from build123d import *

# Parameters (mm, degrees)
SKETCH1_W           = 93.5
SKETCH1_H           = 123
SKETCH1_R           = 6
SKETCH1_W_2         = 57.5
SKETCH1_H_2         = 30
BOSS_EXTRUDE1_DEPTH = 6
SKETCH2_R           = 4.5
SKETCH2_R_2         = 2.1
BOSS_EXTRUDE2_DEPTH = 3
CHAMFER2_SIZE       = 5
SKETCH5_R           = 2.875
CUT_EXTRUDE2_DEPTH  = 3
SKETCH6_R           = 1.625
CUT_EXTRUDE3_DEPTH  = 23
SKETCH7_W           = 5
SKETCH7_H           = 12
SKETCH7_W_2         = 8
SKETCH7_H_2         = 24.8
SKETCH7_R           = 2.1
BOSS_EXTRUDE3_DEPTH = 6
CHAMFER3_SIZE       = 3
CHAMFER3_SIZE2      = 5.196152423
SKETCH9_R           = 2.1
CUT_EXTRUDE5_DEPTH  = 3


with BuildPart() as part:
    # Sketch1 → Boss-Extrude1 (new body)
    with BuildSketch(Plane.XY):
        with Locations((0, 28.5)):
            Rectangle(SKETCH1_W, SKETCH1_H)
        with Locations((0, 60)):
            Circle(SKETCH1_R, mode=Mode.SUBTRACT)
        Rectangle(SKETCH1_W_2, SKETCH1_H_2, mode=Mode.SUBTRACT)
    extrude(amount=BOSS_EXTRUDE1_DEPTH)

    # Sketch2 → Boss-Extrude2 (add)
    # profile 1 of 4: a face of its own
    with BuildSketch(Plane(origin=(0, 0, 0), x_dir=(-1, 0, 0), z_dir=(0, 0, -1))):
        with Locations((34, 21.75)):
            Circle(SKETCH2_R)
        with Locations((34, 21.75)):
            Circle(SKETCH2_R_2, mode=Mode.SUBTRACT)
    # profile 2 of 4: a face of its own
    with BuildSketch(Plane(origin=(0, 0, 0), x_dir=(-1, 0, 0), z_dir=(0, 0, -1))):
        with Locations((-34, -17.25)):
            Circle(SKETCH2_R)
        with Locations((-34, -17.25)):
            Circle(SKETCH2_R_2, mode=Mode.SUBTRACT)
    # profile 3 of 4: a face of its own
    with BuildSketch(Plane(origin=(0, 0, 0), x_dir=(-1, 0, 0), z_dir=(0, 0, -1))):
        with Locations((34, -17.25)):
            Circle(SKETCH2_R)
        with Locations((34, -17.25)):
            Circle(SKETCH2_R_2, mode=Mode.SUBTRACT)
    # profile 4 of 4: a face of its own
    with BuildSketch(Plane(origin=(0, 0, 0), x_dir=(-1, 0, 0), z_dir=(0, 0, -1))):
        with Locations((-34, 21.75)):
            Circle(SKETCH2_R)
        with Locations((-34, 21.75)):
            Circle(SKETCH2_R_2, mode=Mode.SUBTRACT)
    extrude(amount=BOSS_EXTRUDE2_DEPTH)

    # Chamfer2
    chamfer2_edges = [part.edges().sort_by_distance(p)[0] for p in [
        (-46.75, 90, 3),
        (46.75, 90, 3),
        (46.75, -33, 3),
        (-46.75, -33, 3),
    ]]
    chamfer(chamfer2_edges, length=CHAMFER2_SIZE)

    # Sketch5 → Cut-Extrude2 (cut)
    with BuildSketch(Plane.XY.offset(6)):
        with Locations((39.25, -25.5)):
            Circle(SKETCH5_R)
        with Locations((39.25, 82.5)):
            Circle(SKETCH5_R)
        with Locations(Location((-39.25, -25.5, 0), (0, 0, 180))):
            Circle(SKETCH5_R)
        with Locations(Location((-39.25, 82.5, 0), (0, 0, 180))):
            Circle(SKETCH5_R)
    extrude(amount=-CUT_EXTRUDE2_DEPTH, mode=Mode.SUBTRACT)

    # Sketch6 → Cut-Extrude3 (cut)
    with BuildSketch(Plane.XY.offset(3)):
        with Locations((39.25, -25.5)):
            Circle(SKETCH6_R)
        with Locations((-39.25, -25.5)):
            Circle(SKETCH6_R)
        with Locations((-39.25, 82.5)):
            Circle(SKETCH6_R)
        with Locations((39.25, 82.5)):
            Circle(SKETCH6_R)
    extrude(amount=-CUT_EXTRUDE3_DEPTH, mode=Mode.SUBTRACT)

    # Sketch7 → Boss-Extrude3 (add)
    # profile 1 of 2: a face of its own
    with BuildSketch(Plane.XY):
        with Locations((-8, 60)):
            Rectangle(SKETCH7_W, SKETCH7_H)
    # profile 2 of 2: a face of its own
    with BuildSketch(Plane.XY):
        with Locations((9.5, 60)):
            Rectangle(SKETCH7_W_2, SKETCH7_H_2)
        with Locations((8, 51.6)):
            Circle(SKETCH7_R, mode=Mode.SUBTRACT)
        with Locations((8, 68.4)):
            Circle(SKETCH7_R, mode=Mode.SUBTRACT)
    extrude(amount=-BOSS_EXTRUDE3_DEPTH)

    # Chamfer3
    chamfer3_edges = [part.edges().sort_by_distance(p)[0] for p in [
        (-28.75, 0, 6),
        (0, -15, 6),
        (28.75, 0, 6),
        (0, 15, 6),
    ]]
    chamfer3_side = [part.faces().sort_by_distance(p)[0] for p in [
        (0, 33.295685128, 6),
    ]]
    chamfer(chamfer3_edges, length=CHAMFER3_SIZE, length2=CHAMFER3_SIZE2, reference=chamfer3_side[0])

    # Sketch9 → Cut-Extrude5 (cut)
    with BuildSketch(Plane(origin=(0, 0, 0), x_dir=(-1, 0, 0), z_dir=(0, 0, -1))):
        with Locations((30, 75)):
            Circle(SKETCH9_R)
        with Locations((30, 45)):
            Circle(SKETCH9_R)
        with Locations(Location((-30, 45, 0), (0, 0, 180))):
            Circle(SKETCH9_R)
        with Locations(Location((-30, 75, 0), (0, 0, 180))):
            Circle(SKETCH9_R)
    extrude(amount=-CUT_EXTRUDE5_DEPTH, mode=Mode.SUBTRACT)


solid = part.part
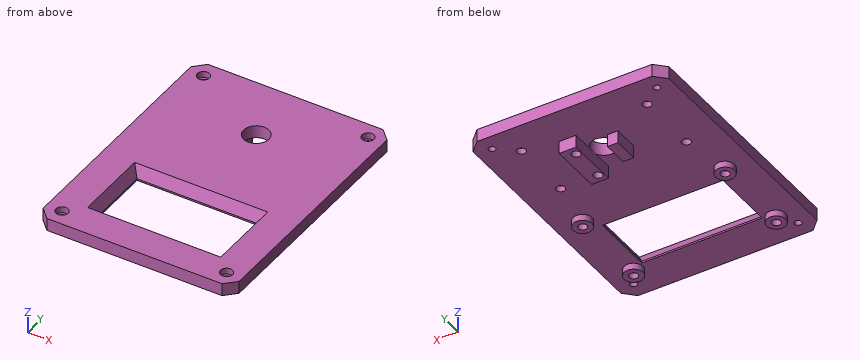
Geometry check sheet. Reference: the model listing, model coordinates, mm. Round coordinates to 2 decimals unless told otherwise and drop trailing zeros. Order: outer loops, then holes, each group sorted by start corner. A loop starts at its lowest first (then second) coordinate and runs counter-clockwise, first axis right, second up. Notation, with made-up numbers: M 25,50 L 48,50 A20 ccw 48,68 Z; hole C -5,9.25 d7. An arc over 180 degrees is marked long. Answer in a Markdown table with one row per item.
(1) Sectioned sample at B-B, the plane y = 60. Record the cut outline in (x, z).
Responses:
| item | result |
|---|---|
| outline | M -46.75,0 L -10.5,0 L -10.5,-6 L -5.5,-6 L -5.5,0 L -6,0 L -6,6 L -46.75,6 Z; M 5.5,-6 L 13.5,-6 L 13.5,0 L 46.75,0 L 46.75,6 L 6,6 L 6,0 L 5.5,0 Z |
(2) Sectioned sample at A-A, the plane x = 20.5. Record the cut outline in (y, z), and give its area (3 significant figures).
Responses:
| item | result |
|---|---|
| outline | M -33,0 L -15,0 L -15,0.8 L -18,6 L -33,6 Z; M 15,0 L 90,0 L 90,6 L 18,6 L 15,0.8 Z |
| area | 542 mm² |
(3) Scan lines: probe 1 along Y at (x, z) = (39.25, 1.25) (3 decimals); probe 2 along Y at (x, z) = (-34, -0.65); probe 3 along Y at (x, z) = (8, -2.25). Record each from-to range of solid material in increasing order. Write a range as from..to.
Responses:
| item | result |
|---|---|
| probe 1 | y = -33..-27.125, -23.875..80.875, 84.125..90 |
| probe 2 | y = -21.75..-19.35, -15.15..-12.75, 17.25..19.65, 23.85..26.25 |
| probe 3 | y = 47.6..49.5, 53.7..66.3, 70.5..72.4 |
(4) Sectioned sample at D-D, the plane y = 82.5. Record the cut outline in (x, z) (3 decimals), and give its area (3 significant figures).
Responses:
| item | result |
|---|---|
| outline | M -46.75,0 L -40.875,0 L -40.875,3 L -42.125,3 L -42.125,6 L -46.75,6 Z; M -37.625,0 L 37.625,0 L 37.625,3 L 36.375,3 L 36.375,6 L -36.375,6 L -36.375,3 L -37.625,3 Z; M 40.875,0 L 46.75,0 L 46.75,6 L 42.125,6 L 42.125,3 L 40.875,3 Z |
| area | 507 mm² |
(5) Go/stop test with flat-tipped pins: P1, Ø7, axis at x = 34.5, y = 22.5, coming from the -Z side; P2, Ø6.5, axis at x = 8, y = 51.6, coming from the -Z side; P3, Ø1.7, axis at x = -38, y = 82.5, coming from the +Z side; P4, Ø1.8, axis at x = 11, z = -2.5, coming from the -Y side. Record where each tip stops, or that it passes through.
Responses:
| item | result |
|---|---|
| P1 | stops at z = -3 |
| P2 | stops at z = -6 |
| P3 | stops at z = 3 |
| P4 | stops at y = 47.6 |
(6) Sectioned sample at C-C, the plane x = 0. Record the cut outline in (y, z), and give its area (3 significant figures).
Responses:
| item | result |
|---|---|
| outline | M -33,0 L -15,0 L -15,0.8 L -18,6 L -33,6 Z; M 15,0 L 54,0 L 54,6 L 18,6 L 15,0.8 Z; M 66,0 L 90,0 L 90,6 L 66,6 Z |
| area | 470 mm² |
